from build123d import *

# Parameters (mm, degrees)
SKETCH1_R                       = 4.7625
BOSS_EXTRUDE1_DEPTH             = 25.4
SKETCH2_OUTSIDE_W               = 17.274
SKETCH2_OUTSIDE_H               = 17.274
SKETCH2_OUTSIDE_W_2             = 4.6482
SKETCH2_OUTSIDE_H_2             = 9.525
CUT_EXTRUDE1_DEPTH              = 5.842
F_3_32_0_09375_DIAMETER_HOLE1_D = 2.38125
CUT_EXTRUDE2_DEPTH              = 27.796665946
TAP_DRILL_FOR_10_24_TAP1_D      = 3.7973
TAP_DRILL_FOR_10_24_TAP1_DEPTH  = 15.875
TAP_DRILL_FOR_10_24_TAP1_TIP    = 1.140824014


with BuildPart() as part:
    # Sketch1 → Boss-Extrude1 (new body)
    with BuildSketch(Plane.XY):
        Circle(SKETCH1_R)
    extrude(amount=BOSS_EXTRUDE1_DEPTH)

    # Sketch2 outside → Cut-Extrude1 (cut)
    with BuildSketch(Plane.XY.offset(25.4)):
        Rectangle(SKETCH2_OUTSIDE_W, SKETCH2_OUTSIDE_H)
        Rectangle(SKETCH2_OUTSIDE_W_2, SKETCH2_OUTSIDE_H_2, mode=Mode.SUBTRACT)
    extrude(amount=-CUT_EXTRUDE1_DEPTH, mode=Mode.SUBTRACT)

    # 3/32 (0.09375) Diameter Hole1 (through all)
    with Locations(Plane.ZY.offset(2.3241)):
        with Locations((22.479, 0)):
            Hole(F_3_32_0_09375_DIAMETER_HOLE1_D / 2)

    # Sketch5 → Cut-Extrude2 (cut, through all)
    with BuildSketch(Plane.ZY.offset(2.3241)):
        with BuildLine():
            Line((22.479, 4.7625), (32.004, 4.7625))
            Line((32.004, 4.7625), (32.004, -4.7625))
            Line((32.004, -4.7625), (22.479, -4.7625))
            ThreePointArc((22.479, -4.7625), (27.2415, 0), (22.479, 4.7625))
        make_face()
    extrude(amount=-CUT_EXTRUDE2_DEPTH, mode=Mode.SUBTRACT)

    # Tap Drill for #10-24 Tap1
    with Locations(Plane(origin=(0, 0, 0), x_dir=(-1, 0, 0), z_dir=(0, 0, -1))):
        with Locations((0, 0)):
            Hole(TAP_DRILL_FOR_10_24_TAP1_D / 2, depth=TAP_DRILL_FOR_10_24_TAP1_DEPTH)
            with Locations((0, 0, -(TAP_DRILL_FOR_10_24_TAP1_DEPTH + TAP_DRILL_FOR_10_24_TAP1_TIP / 2))):  # 118° drill point
                Cone(0, TAP_DRILL_FOR_10_24_TAP1_D / 2, TAP_DRILL_FOR_10_24_TAP1_TIP, mode=Mode.SUBTRACT)


solid = part.part
Input: part model. Units: mm. Frame: model coordinates. A direction names the side the tool comes from. Give positions to 0.01 mm unless a question says otherwise; leave off trailing zeros. Order: outer loops, then holes, each group sorted by start corner. A loop starts at its lowest first (then second) coordinate and runs counter-clockwise, first axis right, second up. Notation, with made-up numbers: M 54,-29.5 L 64,-29.5 A30 ccw 64,8.5 Z; hole C -37.5,40 d10. An arc over 180 degrees is marked long. Answer as a JSON object with one key per item and string values.
1. Reachability of faces 1 (the flat face through (2.324, 0, 24)), 2 (the cylindrical face through (0.03, 0.05, 23.67)), 3 (the flat face through (-2.324, 0, 24)) from +Z, -Z, +X, -X, +Y, -Y: full face, straight path, thin tool, end or side. Return the list, or none.
Result sheet:
{"face 1": "+Z, +X, +Y, -Y", "face 2": "+X, -X", "face 3": "+Z, -X, +Y, -Y"}
2. Cut plane C-C, the plane y = -2.25. Output: boundary loops of the cut face in (x, z), and give its area (3 significant figures).
Result sheet:
{"outline": "M -4.2,0 L 4.2,0 L 4.2,19.56 L 2.32,19.56 L 2.32,25.4 L -2.32,25.4 L -2.32,19.56 L -4.2,19.56 Z", "area": "191 mm²"}
3. First-contact query: P1, Ø1.2, axis at x = -3.5, y = -1.5, coming from the +Z side; P2, Ø2, axis at x = -3, z = 15.5, coming from the +Y side; P3, Ø2.5, axis at x = 3, y = -1.5, coming from the +Z side; P4, Ø1, axis at x = 3.5, z = 17.5, coming from the +Y side. Flat tips, straight axial feed; report the tip coordinate or a pass-through.
Result sheet:
{"P1": "z = 19.56", "P2": "y = 4.32", "P3": "z = 25.4", "P4": "y = 3.7"}
4. Cut plane A-A, the plane z = 23. Output: boundary loops of the cut face in (x, y) (1 decimal), and give its area (3 significant figures).
Result sheet:
{"outline": "M -2.3,-4.2 A4.8 ccw -0.5,-4.7 L 0.5,-4.7 A4.8 ccw 2.3,-4.2 L 2.3,-1.1 L -2.3,-1.1 Z; M -2.3,1.1 L 2.3,1.1 L 2.3,4.2 A4.8 ccw 0.5,4.7 L -0.5,4.7 A4.8 ccw -2.3,4.2 Z", "area": "32.5 mm²"}
5. Pull-direction query (Y, two-part tool) for faces 4 (the cylindrical face through (-1.03, -4.65, 9.47)), 5 (the cylindrical face through (-0.03, 4.37, 24.37)), 6 (the cylindrical face through (1.8, 0.6, 8)); classes: +Y half, -Y half, draft (parallel to the pull), parting line (faces both ways), or undercut.
Result sheet:
{"face 4": "parting line", "face 5": "+Y half", "face 6": "undercut"}
6. Ray query, line 1 (Y direction, x = 0, z = 9.25); line 2 (Z direction, x = 2.75, y = -2.25); line 3 (X direction, y = 0.25, z = 11.5). Return the intervals inside material, ascending. Write a range as [from, to].
Result sheet:
{"line 1": "[-4.76, -1.9], [1.9, 4.76]", "line 2": "[0, 19.56]", "line 3": "[-4.76, -1.88], [1.88, 4.76]"}
7. Cut plane B-B, the plane z = 6.75. Output: boundary loops of the cut face in (x, y) (1 decimal), and give its area (3 significant figures).
Result sheet:
{"outline": "C 0,0 d9.5; hole C 0,0 d3.8", "area": "59.9 mm²"}
8. Cut plane D-D, the plane z = 18.75. Output: boundary loops of the cut face in (x, y) (1 decimal), and give its area (3 significant figures).
Result sheet:
{"outline": "C 0,0 d9.5", "area": "71.3 mm²"}
